Read the model definition and answer for the solid it produces. Units are mm, in the model's axes. Face numbers are marked on the shaded views. A direction names the side the tool comes from. Give positions to 0.01 mm unless a question says otherwise; leave off trailing zeros. Loops run counter-clockwise (first coordinate to the right, second up) from the corner with the lowest first, then second, coordinate; pieces in that order, holes last. Notation, with made-up numbers: (-15.5, 54) -> (29.5, 54) arc R26 cw to (29.5, 78) -> close; hole circle Ø9 at (-17, 89). An arc over 180 degrees is marked (long way). Return JSON: item names as keys, results as strings. Group by question number.
Autodesk Inventor part; units mm, degrees
ref_plane "YZ Plane" through (0, 0, 0) normal (1, 0, 0) x (0, 1, 0)
ref_plane "XZ Plane" through (0, 0, 0) normal (0, 1, 0) x (-1, 0, 0)
ref_plane "XY Plane" through (0, 0, 0) normal (0, 0, 1) x (1, 0, 0)
sketch "Sketch1" plane through (0, 0, 0) normal (0, 1, 0) x (-1, 0, 0)
  line L0 (59.1344, 5.7229) -> (-34.3376, 5.7229)
  line L1 (-34.3376, 5.7229) -> (-34.3376, -46.6011)
  line L2 (-34.3376, -46.6011) -> (59.1344, -46.6011)
  line L3 (59.1344, -46.6011) -> (59.1344, 5.7229)
  point P0 (0, 0)
  dimension "d0" = 52.324
  dimension "d1" = 93.472
extrude "Extrusion1" add sketch "Sketch1" along normal blind 5.08
sketch "Sketch2" plane through (0, 5.08, 0) normal (0, 1, 0) x (1, 0, 0)
  line L0 (34.3376, -5.7229) -> (34.3376, 46.6011)
  line L1 (-59.1344, -5.7229) -> (34.3376, -5.7229)
  line L2 (34.3376, 46.6011) -> (27.9876, 46.6011)
  line L3 (27.9876, 46.6011) -> (27.9876, -5.7229)
  line L4 (27.9876, -5.7229) -> (34.3376, -5.7229)
  line L5 (34.3376, -5.7229) -> (34.3376, 46.6011)
  line L6 (8.9376, 46.6011) -> (2.5876, 46.6011)
  line L7 (2.5876, 46.6011) -> (2.5876, -5.7229)
  line L8 (2.5876, -5.7229) -> (8.9376, -5.7229)
  line L9 (8.9376, -5.7229) -> (8.9376, 46.6011)
  line L10 (34.3376, 46.6011) -> (-59.1344, 46.6011)
  line L11 (-59.1344, 46.6011) -> (-59.1344, -5.7229)
  line L12 (-52.7844, 46.6011) -> (-59.1344, 46.6011)
  line L13 (-59.1344, 46.6011) -> (-59.1344, -5.7229)
  line L14 (-59.1344, -5.7229) -> (-52.7844, -5.7229)
  line L15 (-52.7844, -5.7229) -> (-52.7844, 46.6011)
  point P0 (0, 0)
  dimension "d4" = 6.35
  dimension "d5" = 19.05
  dimension "d6" = 6.35
  dimension "d7" = 6.35
extrude "Extrusion2" add sketch "Sketch2" along normal blind 19.05 contours L1 L3 L2 L0 | L1 L7 L6 L9 | L1 L11 L10 L15
sketch "Sketch3" plane through (0, 24.13, 0) normal (0, 1, 0) x (1, 0, 0)
  line L0 (34.3376, -5.7229) -> (34.3376, 46.6011)
  line L1 (-59.1344, 46.6011) -> (-59.1344, -5.7229)
  line L2 (34.3376, 46.6011) -> (-59.1344, 46.6011)
  line L3 (-59.1344, 46.6011) -> (-59.1344, -5.7229)
  line L4 (-59.1344, -5.7229) -> (34.3376, -5.7229)
  line L5 (34.3376, -5.7229) -> (34.3376, 46.6011)
  point P0 (0, 0)
extrude "Extrusion3" add sketch "Sketch3" along normal blind 6.35
sketch "Sketch4" plane through (0, 30.48, 0) normal (0, 1, 0) x (1, 0, 0)
  point P0 (0, 0)
sketch "Sketch5" plane through (0, 30.48, 0) normal (0, 1, 0) x (1, 0, 0)
  line L0 (-59.1344, -5.7229) -> (34.3376, -5.7229)
  line L1 (-59.1344, -5.7229) -> (-51.5144, -5.7229)
  line L2 (-51.5144, -5.7229) -> (-51.5144, 46.6011)
  line L3 (-51.5144, 46.6011) -> (-59.1344, 46.6011)
  line L4 (-59.1344, 46.6011) -> (-59.1344, -5.7229)
  line L5 (-52.7844, -5.7229) -> (2.5876, -5.7229)
  line L6 (6.5246, -5.7229) -> (14.1446, -5.7229)
  line L7 (14.1446, -5.7229) -> (14.1446, 46.6011)
  line L8 (14.1446, 46.6011) -> (6.5246, 46.6011)
  line L9 (6.5246, 46.6011) -> (6.5246, -5.7229)
  point P0 (0, 0)
  dimension "d12" = 7.62
  dimension "d13" = 7.62
  dimension "d14" = 58.039
extrude "Extrusion4" add sketch "Sketch5" along normal blind 27.94
sketch "Sketch6" plane through (0, 58.42, 0) normal (0, 1, 0) x (1, 0, 0)
  point P0 (0, 0)
sketch "Sketch7" plane through (0, 58.42, 0) normal (0, 1, 0) x (1, 0, 0)
  line L0 (-59.1344, -5.7229) -> (-51.5144, -5.7229)
  line L1 (-51.5144, -5.7229) -> (-51.5144, 46.6011)
  line L2 (-59.1344, -5.7229) -> (-51.5144, -5.7229)
  line L3 (-51.5144, -5.7229) -> (-51.5144, 12.3111)
  line L4 (-51.5144, 12.3111) -> (-59.1344, 12.3111)
  line L5 (-59.1344, 12.3111) -> (-59.1344, -5.7229)
  line L6 (6.5246, -5.7229) -> (6.5246, 46.6011)
  line L7 (14.1446, -5.7229) -> (14.1446, 46.6011)
  line L8 (6.5246, -5.7229) -> (14.1446, -5.7229)
  line L9 (14.1446, -5.7229) -> (14.1446, 12.3111)
  line L10 (14.1446, 12.3111) -> (6.5246, 12.3111)
  line L11 (6.5246, 12.3111) -> (6.5246, -5.7229)
  point P0 (0, 0)
  dimension "d17" = 18.034
extrude "Extrusion5" cut sketch "Sketch7" against normal blind 27.94
sketch "Sketch8" plane through (0, 58.42, 0) normal (0, 1, 0) x (1, 0, 0)
  line L0 (34.3376, 46.6011) -> (-59.1344, 46.6011)
  line L1 (-51.5144, 46.6011) -> (-51.5144, 12.3111)
  line L2 (-59.1344, 46.6011) -> (-51.5144, 46.6011)
  line L3 (-51.5144, 46.6011) -> (-51.5144, 35.1711)
  line L4 (-51.5144, 35.1711) -> (-59.1344, 35.1711)
  line L5 (-59.1344, 35.1711) -> (-59.1344, 46.6011)
  point P0 (0, 0)
  dimension "d20" = 11.43
extrude "Extrusion6" cut sketch "Sketch8" against normal blind 27.94
sketch "Sketch9" plane through (34.3376, 0, -46.6011) normal (0, 0, -1) x (-1, 0, 0)
  line L0 (93.472, 30.48) -> (0, 30.48)
  line L1 (27.813, 30.48) -> (20.193, 30.48)
  line L2 (93.472, 30.48) -> (20.193, 30.48)
  line L3 (20.193, 30.48) -> (20.193, 24.13)
  line L4 (6.35, 24.13) -> (25.4, 24.13)
  line L5 (31.75, 24.13) -> (87.122, 24.13)
  line L6 (25.4, 24.13) -> (31.75, 24.13)
  line L7 (87.122, 5.08) -> (87.122, 24.13)
  line L8 (31.75, 24.13) -> (87.122, 24.13)
  line L9 (93.472, 0) -> (93.472, 30.48)
  line L10 (87.122, 24.13) -> (93.472, 24.13)
  point P0 (34.3376, 0)
extrude "Extrusion7" add sketch "Sketch9" along normal blind 7.62
sketch "Sketch10" plane through (0, 30.48, 0) normal (0, 1, 0) x (1, 0, 0)
  line L0 (14.1446, 46.6011) -> (14.1446, 54.2211)
  line L1 (-59.1344, 54.2211) -> (14.1446, 54.2211)
  line L2 (14.1446, 46.6011) -> (-59.1344, 46.6011)
  line L3 (-59.1344, 46.6011) -> (-59.1344, 54.2211)
  line L4 (-59.1344, 54.2211) -> (14.1446, 54.2211)
  line L5 (14.1446, 54.2211) -> (14.1446, 46.6011)
  point P0 (0, 0)
extrude "Extrusion8" add sketch "Sketch10" along normal blind 27.94
fillet "Fillet1" radius 3.175 4 edges at (2.5876, 5.08, -20.4391) (-52.7844, 5.08, -20.4391) (2.5876, 24.13, -20.4391) (-52.7844, 24.13, -20.4391)
sketch "Sketch11" plane through (-59.1344, 58.42, -12.3111) normal (0, 0, 1) x (1, 0, 0)
  point P0 (59.1344, -58.42)
sketch "Sketch12" plane through (-59.1344, 58.42, -12.3111) normal (0, 0, 1) x (1, 0, 0)
  circle A0 centre (3.81, -6.096) radius 2.54
  line L0 (0, 0) -> (7.62, 0)
  line L1 (0, -27.94) -> (0, 0)
  circle A1 centre (3.81, -21.844) radius 2.54
  line L2 (0, -27.94) -> (7.62, -27.94)
  circle A2 centre (69.469, -6.096) radius 2.54
  line L3 (65.659, 0) -> (73.279, 0)
  line L4 (73.279, 0) -> (73.279, -27.94)
  circle A3 centre (69.469, -21.844) radius 2.54
  line L5 (0, -27.94) -> (93.472, -27.94)
  point P0 (59.1344, -58.42)
  dimension "d29" = 6.096
  dimension "d30" = 3.81
  dimension "d31" = 5.08
  dimension "d32" = 5.08
  dimension "d33" = 3.81
  dimension "d34" = 6.096
  dimension "d35" = 5.08
  dimension "d36" = 6.096
  dimension "d37" = 3.81
  dimension "d38" = 5.08
  dimension "d39" = 3.81
  dimension "d40" = 6.096
hole "Hole1" at (-55.3244, 52.324, -12.3111) at (-55.3244, 36.576, -12.3111) at (10.3346, 52.324, -12.3111) at (10.3346, 36.576, -12.3111) direction (0, 0, -1) diameter 6.35 end through all
sketch "Sketch13" plane through (-59.1344, 0, -46.6011) normal (-1, 0, 0) x (0, 0, 1)
  line L0 (-7.62, 24.13) -> (-7.62, 58.42)
  line L1 (-7.62, 58.42) -> (-7.62, 24.13)
  line L2 (0, 24.13) -> (-7.62, 24.13)
  line L3 (-7.62, 24.13) -> (0, 24.13)
  line L4 (0, 0) -> (0, 24.13)
  line L5 (0, 24.13) -> (0, 0)
  line L6 (0, 0) -> (52.324, 0)
  line L7 (0, 0) -> (52.324, 0)
  line L8 (52.324, 0) -> (52.324, 30.48)
  line L9 (52.324, 0) -> (52.324, 30.48)
  line L10 (34.29, 30.48) -> (34.29, 58.42)
  line L11 (52.324, 30.48) -> (34.29, 30.48)
  line L12 (34.29, 30.48) -> (34.29, 58.42)
  line L13 (34.29, 58.42) -> (11.43, 58.42)
  line L14 (34.29, 58.42) -> (11.43, 58.42)
  line L15 (11.43, 30.48) -> (11.43, 58.42)
  line L16 (11.43, 58.42) -> (11.43, 30.48)
  line L17 (11.43, 30.48) -> (0, 30.48)
  line L18 (11.43, 30.48) -> (0, 30.48)
  line L19 (0, 30.48) -> (0, 58.42)
  line L20 (0, 30.48) -> (0, 58.42)
  line L21 (34.29, 58.42) -> (-7.62, 58.42)
  line L22 (0, 58.42) -> (-7.62, 58.42)
  point P0 (46.6011, 0)
extrude "Extrusion9" add sketch "Sketch13" along normal blind 2.54 contours L0 L21 L19 L17 L15 L13 L10 L11 L8 L6 L4 L2
sketch "Sketch14" plane through (14.1446, 24.13, -46.6011) normal (1, 0, 0) x (0, 0, -1)
  line L0 (-34.29, 34.29) -> (7.62, 34.29)
  line L1 (7.62, 0) -> (7.62, 34.29)
  line L2 (-34.29, 34.29) -> (7.62, 34.29)
  line L3 (7.62, 34.29) -> (7.62, 0)
  line L4 (7.62, 0) -> (-34.29, 0)
  line L5 (-34.29, 0) -> (-34.29, 34.29)
  line L6 (0, 0) -> (7.62, 0)
  line L7 (0, 6.35) -> (-34.29, 6.35)
  line L8 (0, 0) -> (-34.29, 0)
  line L9 (-34.29, 0) -> (-34.29, 6.35)
  line L10 (-34.29, 6.35) -> (0, 6.35)
  line L11 (0, 6.35) -> (0, 0)
  point P0 (-46.6011, -24.13)
extrude "Extrusion10" add sketch "Sketch14" along normal blind 2.54 contours L0 L1 L4 L11 L7 L5
sketch "Sketch15" plane through (0, 5.08, 0) normal (0, 1, 0) x (1, 0, 0)
  point P0 (0, 0)
sketch "Sketch16" plane through (0, 5.08, 0) normal (0, 1, 0) x (1, 0, 0)
  line L0 (34.3376, 46.6011) -> (-61.6744, 46.6011)
  line L1 (-61.6744, -5.7229) -> (34.3376, -5.7229)
  line L2 (-37.502, 46.6011) -> (-31.152, 46.6011)
  line L3 (-31.152, 46.6011) -> (-31.152, -5.7229)
  line L4 (-31.152, -5.7229) -> (-37.502, -5.7229)
  line L5 (-37.502, -5.7229) -> (-37.502, 46.6011)
  line L6 (-19.0447, -5.7229) -> (-12.6947, -5.7229)
  line L7 (-12.6947, -5.7229) -> (-12.6947, 46.6011)
  line L8 (-12.6947, 46.6011) -> (-19.0447, 46.6011)
  line L9 (-19.0447, 46.6011) -> (-19.0447, -5.7229)
  line L10 (-49.6094, -5.7229) -> (-49.6094, 46.6011)
  point P0 (0, 0)
  dimension "d52" = 6.35
  dimension "d53" = 6.35
  dimension "d54" = 12.1073
  dimension "d55" = 12.1073
extrude "Extrusion11" add sketch "Sketch16" along normal blind 25.4 contours L7 L1 L9 L0 | L3 L1 L5 L0
fillet "Fillet2" radius 3.175 1 edges at (-37.502, 5.08, -20.4391)
fillet "Fillet3" radius 3.175 1 edges at (-19.0447, 5.08, -20.4391)
fillet "Fillet4" radius 3.175 1 edges at (-31.152, 24.13, -20.4391)
fillet "Fillet5" radius 3.175 1 edges at (-12.6947, 24.13, -20.4391)
fillet "Fillet6" radius 3.175 1 edges at (-12.6947, 5.08, -20.4391)
fillet "Fillet7" radius 3.175 1 edges at (-31.152, 5.08, -20.4391)
fillet "Fillet8" radius 3.175 1 edges at (-37.502, 24.13, -20.4391)
fillet "Fillet9" radius 3.175 1 edges at (-19.0447, 24.13, -20.4391)
sketch "Sketch17" plane through (27.9876, 5.08, -46.6011) normal (-1, 0, 0) x (0, 0, 1)
  line L0 (0, 19.05) -> (-7.62, 19.05)
  line L1 (52.324, 0) -> (0, 0)
  line L2 (0, 19.05) -> (52.324, 19.05)
  line L3 (52.324, 19.05) -> (52.324, 0)
  line L4 (52.324, 0) -> (0, 0)
  line L5 (0, 0) -> (0, 19.05)
  point P0 (46.6011, -5.08)
extrude "Extrusion12" cut sketch "Sketch17" against normal blind 0.635
sketch "Sketch18" plane through (8.9376, 5.08, 5.7229) normal (1, 0, 0) x (0, 0, -1)
  line L0 (52.324, 15.875) -> (52.324, 19.05)
  line L1 (0, 0) -> (52.324, 0)
  line L2 (52.324, 19.05) -> (0, 19.05)
  line L3 (0, 19.05) -> (0, 0)
  line L4 (0, 0) -> (52.324, 0)
  line L5 (52.324, 0) -> (52.324, 19.05)
  point P0 (5.7229, -5.08)
extrude "Extrusion13" cut sketch "Sketch18" against normal blind 0.635
sketch "Sketch19" plane through (0, 24.13, 0) normal (0, -1, 0) x (1, 0, 0)
  line L0 (28.6226, 5.7229) -> (28.6226, -46.6011)
  line L1 (-61.6744, 5.7229) -> (34.3376, 5.7229)
  line L2 (28.6226, -46.6011) -> (8.1284, -46.6011)
  line L3 (8.1284, -46.6011) -> (8.1284, 5.7229)
  line L4 (8.1284, 5.7229) -> (28.6226, 5.7229)
  line L5 (28.6226, 5.7229) -> (28.6226, -46.6011)
  point P0 (0, 0)
extrude "Extrusion14" cut sketch "Sketch19" against normal blind 0.635
sketch "Sketch20" plane through (0, 5.08, 0) normal (0, 1, 0) x (1, 0, 0)
  line L0 (28.6226, -5.7229) -> (28.6226, 46.6011)
  line L1 (16.6846, 46.6011) -> (8.3026, 46.6011)
  line L2 (28.6226, -5.7229) -> (8.3026, -5.7229)
  line L3 (8.3026, -5.7229) -> (8.3026, 46.6011)
  line L4 (8.3026, 46.6011) -> (28.6226, 46.6011)
  line L5 (28.6226, 46.6011) -> (28.6226, -5.7229)
  point P0 (0, 0)
extrude "Extrusion15" cut sketch "Sketch20" against normal blind 0.635
sketch "Sketch21" plane through (0, 24.13, 0) normal (0, -1, 0) x (1, 0, 0)
  line L0 (16.6846, -46.6011) -> (16.6846, -54.2211)
  line L1 (-49.6094, -46.6011) -> (-61.6744, -46.6011)
  line L2 (16.6846, -54.2211) -> (-61.6744, -54.2211)
  line L3 (-61.6744, -54.2211) -> (-61.6744, -46.6011)
  line L4 (-61.6744, -46.6011) -> (16.6846, -46.6011)
  line L5 (16.6846, -46.6011) -> (16.6846, -54.2211)
  point P0 (0, 0)
extrude "Extrusion16" cut sketch "Sketch21" against normal blind 0.635
properties part number "Nov 21 holder for arm server (resized hole)"
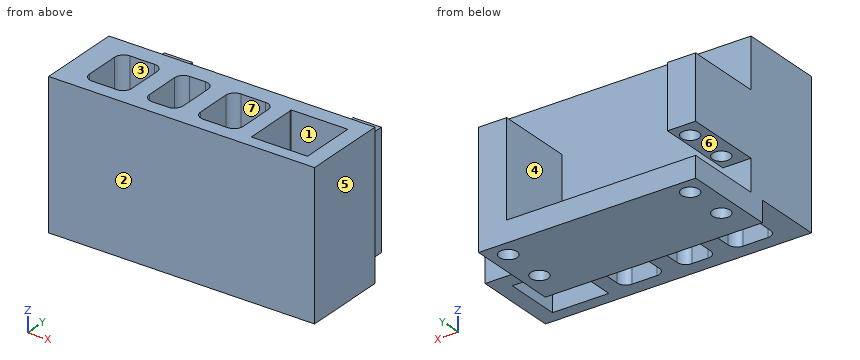
1. Section A-A on y = 32 is taken. Determine the outline of the cut face in (x, z).
2. Determine the mould class of the marked faces 5, 6 and 7 for opening direction X: pulls with the +X half, pulls with the -X half, needs draft (parallel to the pull), parting line crosses it, or undercut.
3. Section D-D on y = 51 is taken. Determine the outline of the cut face in (x, z), then the cut area to 3 significant figures.
4. Section C-C on z = -8 is taken. State how many separate pieces and enclosed holes the cut face has, then the cut area to 3 significant figures.
5. Section B-B on x = -26.5 is taken. Determine the outline of the cut face in (y, z) (3 decimals), then the cut area to 3 significant figures.
6. Which of the six approach directions +Z, -Z, +X, -X, +Y, -Y give full straight-line access (tool end or side, diameter ignored) to the marked faces 1, 2, 3 and 4?
7. Flat-ended cylindrical pins translate along their axes: pin 1 Ø6 at (y, z) = (46, -40.5) entering from +X; pin 2 Ø5 at (x, y) = (-2, 15) entering from -Z; pin 3 Ø1 at (x, z) = (-25.5, -27) entering from +Y; pin 4 Ø8 at (x, y) = (20, 52.5) entering from +Z. Find the tip coordinate at first contact, or state that the pin passes through.
8. Straight lines are drawn through the part: line 1 (X direction, y = 12, z = -19); line 2 (Y direction, x = 10, z = -22.5) (3 decimals); line 3 (Y direction, x = -48.5, z = -41). For each, find the intervals that lie inside material, in ascending order. Write a range as from..to.
Completed:
{
 "1": {"outline": "(-61.67, -54.22) -> (16.68, -54.22) -> (16.68, -12.31) -> (6.52, -12.31) -> (6.52, -46.6) -> (-61.67, -46.6) -> close; (-61.67, -35.17) -> (-51.51, -35.17) -> (-51.51, -12.31) -> (-61.67, -12.31) -> close"},
 "2": {"face 5": "pulls with the +X half", "face 6": "needs draft", "face 7": "undercut"},
 "3": {"outline": "(-61.67, -54.22) -> (-58.21, -54.22) -> (-58.21, -46.6) -> (-61.67, -46.6) -> close; (-61.67, -35.17) -> (-58.21, -35.17) -> (-58.21, -12.31) -> (-61.67, -12.31) -> close; (-52.44, -54.22) -> (7.45, -54.22) -> (7.45, -12.31) -> (6.52, -12.31) -> (6.52, -46.6) -> (-52.44, -46.6) -> close; (-52.44, -35.17) -> (-51.51, -35.17) -> (-51.51, -12.31) -> (-52.44, -12.31) -> close; (13.22, -54.22) -> (16.68, -54.22) -> (16.68, -12.31) -> (13.22, -12.31) -> close", "area": "760 mm²"},
 "4": {"separate pieces": "1", "enclosed holes": "4", "area": "1,730 mm²"},
 "5": {"outline": "(0, -46.601) -> (5.08, -46.601) -> (5.08, 5.723) -> (0, 5.723) -> close; (24.13, -46.601) -> (24.765, -46.601) -> (24.765, -54.221) -> (58.42, -54.221) -> (58.42, -46.601) -> (30.48, -46.601) -> (30.48, 5.723) -> (24.13, 5.723) -> close", "area": "855 mm²"},
 "6": {"face 1": "-Z", "face 2": "+Z, -Z, +X, -X, -Y", "face 3": "+Z, -Z", "face 4": "+Z, +Y"},
 "7": {"pin 1": "stops at x = 16.68", "pin 2": "passes through", "pin 3": "stops at y = 30.48", "pin 4": "stops at z = -12.31"},
 "8": {"line 1": "x = -61.67..-52.78, -37.5..-31.15, -19.04..-12.69, 2.59..8.3, 28.62..34.34", "line 2": "y = 0..4.445, 24.765..33.419, 39.733..49.167, 55.481..58.42", "line 3": "y = 0..5.08, 24.13..30.48"}
}
